Geometry: final body of the model. Coordinates: model frame, mm. Round coordinates to 2 decimals unless told otherwise and drop trailing zeros. Order: outer loops, then holes, each group sorted by start corner. A loop starts at its lowest first (then second) coordinate and runs counter-clockwise, first axis right, second up. Notation, with made-up numbers: M 32.5,71 L 78.5,71 A15 ccw 78.5,84 Z; hole C 89,82 d11. An arc over 180 degrees is marked long. Return JSON: item names as keys, results as strings. Group by question number.
Q1. Cut plane B-B on x = 0. Output: boundary loops of the cut face in (y, z), and give its area (3 significant figures).
Q2. Ray query, probe 1 along X at (y, z) = (2.5, 0); probe 2 along X at (y, z) = (1.75, 1); probe 3 along X at (y, z) = (2.75, 4.5). Return the intervals inside material, ascending.
Q3. Contact query for flat-ended pins moving along their axis: pin 1 (2 mm diameter, centred on x = 10.5, z = 3.5, fed in from +Y); pin 2 (1 mm diameter, centred on x = -22.5, y = 0.5, fed in from +Z); pin 3 (3 mm diameter, centred on y = 3, z = 2.5, fed in from -X); pin 4 (1 mm diameter, centred on y = 3, z = 7, fed in from +X). Output: stop coordinate, or through.
Q4. Cut plane D-D on z = 7.5. Output: boundary loops of the cut face in (x, y).
Q5. Cut plane C-C on y = 3.1. Output: boundary loops of the cut face in (x, z), and give its area (3 significant figures).
Q6. Mould query, pull axis Z, two halves, no side actions, for faces 1 (the face through (-2, 0, -4)), 2 (the face through (-20.97, 2.71, -2.1)), 3 (the face through (-9.36, 2.71, -2.96)). Classes: released by +Z, released by -Z, zero draft, split by the parting line, or undercut.
Q7. Cut plane A-A on z = 0. Output: boundary loops of the cut face in (x, y).
```python
from build123d import *

# Parameters (mm, degrees)
SCHIZZO1_R                   = 4
ESTRUSIONE_ESTRUSIONE1_DEPTH = 5.5


with BuildPart() as part:
    # Schizzo1 → Estrusione-Estrusione1 (new body)
    with BuildSketch(Plane(origin=(0, 0, 0), x_dir=(1, 0, 0), z_dir=(0, 1, 0))):
        with BuildLine():
            Line((-31.25, 1), (-10.389548196, 3.231490655))
            ThreePointArc((-10.389548196, 3.231490655), (-9.349630999, 2.954475369), (-8.762875038, 2.0523209))
            ThreePointArc((-8.762875038, 2.0523209), (-0.533351916, -8.98418253), (8.944145279, 1.001131971))
            Line((8.944145279, 1.001131971), (27.25, 6))
            ThreePointArc((27.25, 6), (28.75, 7.5), (27.25, 9))
            Line((27.25, 9), (-27.25, 9))
            Line((-27.25, 9), (-31.25, 1))
        make_face()
        with Locations(Location((0, 0, 0), (0, 0, 270))):
            Circle(SCHIZZO1_R, mode=Mode.SUBTRACT)
    extrude(amount=ESTRUSIONE_ESTRUSIONE1_DEPTH)


solid = part.part
```
Result sheet:
{
 "1": {"outline": "M 0,-9 L 5.5,-9 L 5.5,-4 L 0,-4 Z; M 0,4 L 5.5,4 L 5.5,9 L 0,9 Z", "area": "55.0 mm²"},
 "2": {"probe 1": "x = -9 to -4, 4 to 9", "probe 2": "x = -8.94 to -3.87, 3.87 to 8.94", "probe 3": "x = -7.79 to 7.79"},
 "3": {"pin 1": "passes through", "pin 2": "stops at z = -1.88", "pin 3": "stops at x = -8.94", "pin 4": "stops at x = 6.22"},
 "4": {"outline": "M -4.97,0 L 4.97,0 L 4.97,5.5 L -4.97,5.5 Z"},
 "5": {"outline": "M -31.25,-1 L -27.25,-9 L 27.25,-9 A1.5 ccw 27.25,-6 L 8.94,-1 A9 ccw long -8.76,-2.05 A1.5 cw -10.39,-3.23 Z; hole C 0,0 d8", "area": "478 mm²"},
 "6": {"face 1": "zero draft", "face 2": "released by +Z", "face 3": "undercut"},
 "7": {"outline": "M -9,0 L -4,0 L -4,5.5 L -9,5.5 Z; M 4,0 L 9,0 L 9,5.5 L 4,5.5 Z"}
}
